Verification items for the finished model (mm, model axes). A direction names the side the tool comes from. Round coordinates to 2 decimals unless told otherwise and drop trailing zeros. Loops run counter-clockwise (first coordinate to the right, second up) from the corner with the lowest first, then second, coordinate; pieces in that order, holes last.
from build123d import *

# Parameters (mm, degrees)
BOSS_EXTRUDE1_DEPTH = 20
SKETCH2_R           = 2.25
CUT_EXTRUDE1_DEPTH  = 40


with BuildPart() as part:
    # Sketch1 → Boss-Extrude1 (new, symmetric)
    with BuildSketch(Plane.XY):
        Polygon((-150, 7.75), (-150, -7.75), (150, -7.75), (150, 7.75), (20, 7.75), (20, 0.25), (-20, 0.25), (-20, 7.75), align=None)
    extrude(amount=BOSS_EXTRUDE1_DEPTH, both=True)

    # Sketch2 → Cut-Extrude1 (cut)
    with BuildSketch(Plane(origin=(0, 0.25, 0), x_dir=(1, 0, 0), z_dir=(0, 1, 0))):
        with Locations(Location((15.015, 15, 0), (0, 0, 270))):
            Circle(SKETCH2_R)
        with Locations(Location((-15.015, 15, 0), (0, 0, 180))):
            Circle(SKETCH2_R)
        with Locations(Location((15.015, -15, 0), (0, 0, 180))):
            Circle(SKETCH2_R)
        with Locations(Location((-15.015, -15, 0), (0, 0, 270))):
            Circle(SKETCH2_R)
        Polygon((0, -9.814954576), (8.5, -4.907477288), (8.5, 4.907477288), (0, 9.814954576), (-8.5, 4.907477288), (-8.5, -4.907477288), align=None)
    extrude(amount=-CUT_EXTRUDE1_DEPTH, mode=Mode.SUBTRACT)


solid = part.part
1. Section check A-A (y = 3.75). Enter the section's corners in (x, z), then the cut area to 3 significant figures.
2. Tool access check on faces 1 (the face through (-9, 0.25, 0)), 2 (the face through (4.191, -3.694, 7.396)), 3 (the face through (-2, 0, -20)). Record the directions out of +Z, -Z, +X, -X, +Y, -Y that give a thin tool (end or side, any length) a straight path to the whole face; none if there is none.
3. Release check for a two-part mould opening along Z. For faces 4 (the face through (4.309, -3.694, -7.327)), 5 (the face through (-2, -7.75, 9)), 6 (the face through (-2, 0, 20)) record: released by +Z, released by -Z, zero draft, split by the parting line, or undercut.
4. Scan lines: L1, parallel to X at y = -6.75, z = -13.5; L2, parallel to X at y = 6.5, z = -8.5; L3, parallel to X at y = -2.75, z = 0. Record each from-to range of solid material in increasing order.
Taken from the geometry:
1. outline: (-150, -20) - (-20, -20) - (-20, 20) - (-150, 20) - close; (20, -20) - (150, -20) - (150, 20) - (20, 20) - close
1. area: 10,400 mm2
2. face 1: +Z, -Z, +Y
2. face 2: +Y, -Y
2. face 3: -Z, +X, -X, +Y, -Y
3. face 4: undercut
3. face 5: zero draft
3. face 6: released by +Z
4. L1: x = -150 to -16.69, -13.34 to 13.34, 16.69 to 150
4. L2: x = -150 to -20, 20 to 150
4. L3: x = -150 to -8.5, 8.5 to 150
